```python
from build123d import *

# Parameters (mm, degrees)
SKETCH1_R           = 0.5
BOSS_EXTRUDE1_DEPTH = 2
FILLET1_R           = 30
FILLET5_R           = 100
FILLET2_R           = 10
FILLET3_R           = 1
FILLET4_R           = 5


with BuildPart() as part:
    # Sketch1 → Boss-Extrude1 (new body)
    with BuildSketch(Plane(origin=(0, 0, 0), x_dir=(0, 1, 0), z_dir=(0, 0, 1))):
        Polygon((-89.468095407, -10.44451917), (-68.806810142, -7.332792233), (-70.103747412, 7.491268603), (-47.5, 9.468840255), (-47.5, 22.5), (-28.5, 22.5), (-28.5, 12.5), (-9.5, 12.5), (-9.5, 9.5), (9.5, 9.5), (9.5, 3), (30.24, 3), (30.24, -33.48), (17.635245125, -53.075343018), (14.662990289, -71.841421489), (-48.241456697, -61.878335859), (-80.979250129, -66.808865222), align=None)
        with Locations(Location((-56.5, -39, 0), (0, 0, 270))):
            Circle(SKETCH1_R, mode=Mode.SUBTRACT)
        with Locations(Location((-73, -56, 0), (0, 0, 270))):
            Circle(SKETCH1_R, mode=Mode.SUBTRACT)
        with Locations(Location((0, 0, 0), (0, 0, 270))):
            Circle(SKETCH1_R, mode=Mode.SUBTRACT)
        with Locations(Location((-38, 13, 0), (0, 0, 270))):
            Circle(SKETCH1_R, mode=Mode.SUBTRACT)
        with Locations(Location((-19, 3, 0), (0, 0, 270))):
            Circle(SKETCH1_R, mode=Mode.SUBTRACT)
        with Locations(Location((12, 0, 0), (0, 0, 270))):
            Circle(SKETCH1_R, mode=Mode.SUBTRACT)
        with Locations(Location((-12, -58, 0), (0, 0, 270))):
            Circle(SKETCH1_R, mode=Mode.SUBTRACT)
        with Locations(Location((0, -19, 0), (0, 0, 270))):
            Circle(SKETCH1_R, mode=Mode.SUBTRACT)
        with Locations(Location((-19, -16, 0), (0, 0, 270))):
            Circle(SKETCH1_R, mode=Mode.SUBTRACT)
        with Locations(Location((-38, -6, 0), (0, 0, 270))):
            Circle(SKETCH1_R, mode=Mode.SUBTRACT)
        with Locations(Location((0, -38, 0), (0, 0, 270))):
            Circle(SKETCH1_R, mode=Mode.SUBTRACT)
        with Locations(Location((-19, -35, 0), (0, 0, 270))):
            Circle(SKETCH1_R, mode=Mode.SUBTRACT)
        with Locations(Location((-38, -25, 0), (0, 0, 270))):
            Circle(SKETCH1_R, mode=Mode.SUBTRACT)
        with Locations(Location((-58.155959112, -20.072300736, 0), (0, 0, 270))):
            Circle(SKETCH1_R, mode=Mode.SUBTRACT)
        with Locations(Location((-59.811918224, -1.144601473, 0), (0, 0, 270))):
            Circle(SKETCH1_R, mode=Mode.SUBTRACT)
        with Locations(Location((-75.829615093, -37.211884649, 0), (0, 0, 270))):
            Circle(SKETCH1_R, mode=Mode.SUBTRACT)
        with Locations(Location((-78.659230186, -18.423769299, 0), (0, 0, 270))):
            Circle(SKETCH1_R, mode=Mode.SUBTRACT)
        with Locations(Location((6.766078471, -60.972254836, 0), (0, 0, 270))):
            Circle(SKETCH1_R, mode=Mode.SUBTRACT)
    extrude(amount=BOSS_EXTRUDE1_DEPTH)

    # Fillet1
    fillet1_edges = [part.edges().sort_by_distance(p)[0] for p in [
        (53.075343018, 17.635245125, 1),
    ]]
    fillet(fillet1_edges, radius=FILLET1_R)

    # Fillet5
    fillet5_edges = [part.edges().sort_by_distance(p)[0] for p in [
        (61.878335859, -48.241456697, 1),
    ]]
    fillet(fillet5_edges, radius=FILLET5_R)

    # Fillet2
    fillet2_edges = [part.edges().sort_by_distance(p)[0] for p in [
        (33.48, 30.24, 1),
    ]]
    fillet(fillet2_edges, radius=FILLET2_R)

    # Fillet3
    fillet3_edges = [part.edges().sort_by_distance(p)[0] for p in [
        (10.44451917, -89.468095407, 1),
        (-7.491268603, -70.103747412, 1),
        (-22.5, -47.5, 1),
        (-22.5, -28.5, 1),
        (-12.5, -9.5, 1),
        (-9.5, -9.5, 1),
        (-9.5, 9.5, 1),
        (-3, 30.24, 1),
        (71.841421489, 14.662990289, 1),
        (66.808865222, -80.979250129, 1),
    ]]
    fillet(fillet3_edges, radius=FILLET3_R)

    # Fillet4
    fillet4_edges = [part.edges().sort_by_distance(p)[0] for p in [
        (7.332792233, -68.806810142, 1),
        (-9.468840255, -47.5, 1),
        (-12.5, -28.5, 1),
        (-3, 9.5, 1),
    ]]
    fillet(fillet4_edges, radius=FILLET4_R)


solid = part.part
```
Part model, mm, in its own coordinate system. A direction names the side the tool comes from. Round coordinates to 2 decimals unless told otherwise and drop trailing zeros. Loops run counter-clockwise (first coordinate to the right, second up) from the corner with the lowest first, then second, coordinate; pieces in that order, holes last. Notation, with made-up numbers: (22, 40.5) -> (64, 40.5) arc R30 cw to (64, 78.5) -> close; hole circle Ø7 at (17.5, 23). An arc over 180 degrees is marked (long way). Use a Markdown table: item, result.
1) Tool access for faces 4 (the cylindrical face through (6.22, -70.3, 1.01)), 5 (the flat face through (65.402, -71.639, 0.986)): list every direction of +Z, -Z, +X, -X, +Y, -Y with a clear straight run to the whole face (end or side of a thin tool).
The answers:
| item | result |
|---|---|
| face 4 | +Z, -Z, -Y |
| face 5 | +Z, -Z, +X |
2) Cut at B-B, the plane y = 4. List the corners of the cut face in (x, z).
The answers:
| item | result |
|---|---|
| outline | (-9.5, 0) -> (70.15, 0) -> (70.15, 2) -> (-9.5, 2) -> close |
3) Probe line 1 (X direction, y = -38, z = 0.8); line 2 (Y direction, x = 6, z = 1.3); line 3 (Y direction, x = 17, z = 1.05). List the from-to ranges inside material, lowest first. Write a range as [from, to].
The answers:
| item | result |
|---|---|
| line 1 | x = [-22.5, -13.5], [-12.5, 5.5], [6.5, 24.5], [25.5, 63.63] |
| line 2 | y = [-70.13, -38.5], [-37.5, 30.24] |
| line 3 | y = [-88.48, 30.24] |
4) Pull direction Y, two halves, no side cores. Call faces 1 (the flat face through (24, -29, 2)), 2 (the flat face through (39.007, -85.166, 0.986)), 3 (the flat face through (68.04, -9.33, 0.99)): pulls with the +Y half, pulls with the -Y half, needs draft (parallel to the pull), parting line crosses it, or undercut.
The answers:
| item | result |
|---|---|
| face 1 | needs draft |
| face 2 | pulls with the -Y half |
| face 3 | undercut |
5) Drop flat-ended pins along their axis: pin 1 Ø0.5 at (x, z) = (-11, 1.5) entering from +Y; pin 2 Ø1 at (y, z) = (19.5, 0.5) entering from -X; pin 3 Ø0.6 at (y, z) = (-16.5, 1) entering from -X. Give the stop position or say it passes through.
The answers:
| item | result |
|---|---|
| pin 1 | stops at y = -9.5 |
| pin 2 | stops at x = -3 |
| pin 3 | stops at x = -12.5 |
6) Cut at A-A, the plane z = 1.1. State how many separate pieces and enclosed holes the cut face has, and give its area (3 significant figures).
The answers:
| item | result |
|---|---|
| separate pieces | 1 |
| enclosed holes | 18 |
| area | 8,300 mm2 |
